Check sheet for the modelled part. Datum: model origin and axes. Units: mm. A direction names the side the tool comes from. Coordinates: 2 decimals unless noted, no trailing zeros. Loops run counter-clockwise (first coordinate to the right, second up) from the corner with the lowest first, then second, coordinate; pieces in that order, holes last. Notation, with made-up numbers: (58, 59) -> (72, 59) arc R11 ccw to (72, 63) -> close; hole circle Ø10 at (68, 67). An arc over 180 degrees is marked (long way). Use CSV: the item, a comma, the result in double quotes. Start each with the question number.
1. Release check for a two-part mould opening along Z. For faces 1 (the face through (33, 0, 0)), 2 (the face through (0.773, 0.626, 48.813)), 3 (the face through (0, 0, 32)), 4 (the face through (0.77, -12.61, 27.48)) record: pulls with the +Z half, pulls with the -Z half, needs draft (parallel to the pull), parting line crosses it, or undercut.
2. Gauge pin test, flat ends, axial feed: pin 1 (11.5 mm diameter, centred on y = 5, z = 28, fed in from +X); pin 2 (12 mm diameter, centred on x = 34.5, y = 6, fed in from +Z); pin 3 (3.5 mm diameter, centred on x = 50.8, y = 0, fed in from +Z). Record the tip position at first contact, or that the pin passes through.
3. Sectioned sample at B-B, the plane x = 25.4. Record the cut outline in (y, z).
4. Thickness scan on L1, parallel to Y at x = 25.4, z = 1; L2, parallel to X at y = -2, z = 16.5. Record the ranges inside material, lowest first.
5. Sectioned sample at C-C, the plane y = 12.7. Record the cut outline in (x, z), and give its area (3 significant figures).
6. Set-up check for faces 5 (the face through (1.524, 0, 33)), 6 (the face through (0.77, 12.79, 27.48)): record each of +Z, -Z, +X, -X, +Y, -Y from which the full face is reachable in a straight line by a thin tool's end or side.
7. Sectioned sample at D-D, the plane z = 25.4. Record the cut outline in (x, y).
8. Sectioned sample at A-A, the plane z = 50.8. Record the cut outline in (x, y), and give its area (3 significant figures).
```python
from build123d import *

# Parameters (mm, degrees)
EXTRUDE_THIN1_START = -19.05
EXTRUDE_THIN1_DEPTH = 38.1
SKETCH4_R           = 2.0828
EXTRUDE3_DEPTH      = 91.75338603


# Read off the part's stored shape, not the designer's step: Extrude-Thin1
with BuildPart() as part:
    # Extrude-Thin1 outline → Extrude-Thin1 (new body)
    with BuildSketch(Plane(origin=(0, 0, 0), x_dir=(1, 0, 0), z_dir=(0, 1, 0)).offset(EXTRUDE_THIN1_START)):
        with BuildLine():
            Line((2.286, -1.524), (63.5, -1.524))
            Line((63.5, -1.524), (63.5, 0))
            Line((63.5, 0), (2.286, 0))
            ThreePointArc((2.286, 0), (0.669553898, -0.669553898), (0, -2.286))
            Line((0, -2.286), (0, -63.5))
            Line((0, -63.5), (1.524, -63.5))
            Line((1.524, -63.5), (1.524, -2.286))
            ThreePointArc((1.524, -2.286), (1.747184633, -1.747184633), (2.286, -1.524))
        make_face()
    extrude(amount=EXTRUDE_THIN1_DEPTH)

    # Sketch4 → Extrude3 (cut, through all)
    with BuildSketch(Plane(origin=(1.524, 0, 0), x_dir=(0, 0, -1), z_dir=(1, 0, 0))):
        with Locations((-50.8, 0)):
            Circle(SKETCH4_R)
        with Locations((-25.4, 12.7)):
            Circle(SKETCH4_R)
        with Locations((-25.4, -12.7)):
            Circle(SKETCH4_R)
    extrude3 = extrude(amount=-EXTRUDE3_DEPTH, mode=Mode.SUBTRACT)

    # Mirror1: Extrude3 across plane
    add(extrude3.mirror(Plane(origin=(0, 0, 0), x_dir=(0.7071067811865465, 0, 0.7071067811865486), z_dir=(-0.7071067811865488, 0, 0.7071067811865464))), mode=Mode.SUBTRACT)


solid = part.part
```
Completed:
1,face 1,"pulls with the -Z half"
1,face 2,"undercut"
1,face 3,"needs draft"
1,face 4,"undercut"
2,pin 1,"x = 1.52"
2,pin 2,"z = 1.52"
2,pin 3,"through"
3,outline,"(-19.05, 0) -> (-14.78, 0) -> (-14.78, 1.52) -> (-19.05, 1.52) -> close; (-10.62, 0) -> (10.62, 0) -> (10.62, 1.52) -> (-10.62, 1.52) -> close; (14.78, 0) -> (19.05, 0) -> (19.05, 1.52) -> (14.78, 1.52) -> close"
4,L1,"-19.05 to -14.78, -10.62 to 10.62, 14.78 to 19.05"
4,L2,"0 to 1.52"
5,outline,"(0, 2.29) arc R2.29 ccw to (2.29, 0) -> (23.32, 0) -> (23.32, 1.52) -> (2.29, 1.52) arc R0.76 cw to (1.52, 2.29) -> (1.52, 23.32) -> (0, 23.32) -> close; (0, 27.48) -> (1.52, 27.48) -> (1.52, 63.5) -> (0, 63.5) -> close; (27.48, 0) -> (63.5, 0) -> (63.5, 1.52) -> (27.48, 1.52) -> close"
5,area,"178 mm²"
6,face 5,"+Z, +X, +Y, -Y"
6,face 6,"+X, -X"
7,outline,"(0, -19.05) -> (1.52, -19.05) -> (1.52, -14.78) -> (0, -14.78) -> close; (0, -10.62) -> (1.52, -10.62) -> (1.52, 10.62) -> (0, 10.62) -> close; (0, 14.78) -> (1.52, 14.78) -> (1.52, 19.05) -> (0, 19.05) -> close"
8,outline,"(0, -19.05) -> (1.52, -19.05) -> (1.52, -2.08) -> (0, -2.08) -> close; (0, 2.08) -> (1.52, 2.08) -> (1.52, 19.05) -> (0, 19.05) -> close"
8,area,"51.7 mm²"
